```python
from build123d import *

# Parameters (mm, degrees)
SKETCH1_R               = 23.8125
SKETCH1_R_2             = 21.2725
BOSS_EXTRUDE1_DEPTH     = 27.94
SKETCH2_W               = 24.892
SKETCH2_H               = 1.27
SKETCH5_R               = 21.2725
BOSS_EXTRUDE2_DEPTH     = 0.635
CUT_EXTRUDE2_DEPTH      = 37.706625253
CUT_EXTRUDE2_DEPTH_BACK = 37.706625253
SKETCH7_R               = 5.08
BOSS_EXTRUDE7_DEPTH     = 23.495
CUT_EXTRUDE3_DEPTH      = 19.05


with BuildPart() as part:
    # Sketch1 → Boss-Extrude1 (new body)
    with BuildSketch(Plane.XY):
        Circle(SKETCH1_R)
        Circle(SKETCH1_R_2, mode=Mode.SUBTRACT)
    extrude(amount=BOSS_EXTRUDE1_DEPTH)

    # Sketch2 → Cut-Revolve2 (revolve, cut)
    with BuildSketch(Plane(origin=(0, 0, 0), x_dir=(0, 0, -1), z_dir=(1, 0, 0))):
        with Locations((-13.97, 23.1775)):
            Rectangle(SKETCH2_W, SKETCH2_H)
    revolve(axis=Axis((0, 0, 0), (0, 0, 1)), mode=Mode.SUBTRACT)

    # Sketch5 → Boss-Extrude2 (add, symmetric)
    with BuildSketch(Plane.XY.offset(13.97)):
        Circle(SKETCH5_R)
    extrude(amount=BOSS_EXTRUDE2_DEPTH, both=True)

    # Sketch6 → Cut-Extrude2 (cut, two sides: drawn at the far end of the back side and taken through both)
    with BuildSketch(Plane.XY.offset(14.605).offset(-CUT_EXTRUDE2_DEPTH_BACK)):
        with BuildLine():
            Line((0, 5.08), (0, 20.076289255))
            ThreePointArc((0, 20.076289255), (6.203914564, 19.093685719), (11.800546745, 16.242059191))
            Line((11.800546745, 16.242059191), (2.985949082, 4.109806331))
            ThreePointArc((2.985949082, 4.109806331), (1.569806331, 4.831367103), (0, 5.08))
        make_face()
        with BuildLine():
            Line((4.831367103, 1.569806331), (19.093685719, 6.203914564))
            ThreePointArc((19.093685719, 6.203914564), (20.076289255, 0), (19.093685719, -6.203914564))
            Line((19.093685719, -6.203914564), (4.831367103, -1.569806331))
            ThreePointArc((4.831367103, -1.569806331), (5.08, 0), (4.831367103, 1.569806331))
        make_face()
        with BuildLine():
            Line((2.985949082, -4.109806331), (11.800546745, -16.242059191))
            ThreePointArc((11.800546745, -16.242059191), (6.203914564, -19.093685719), (0, -20.076289255))
            Line((0, -20.076289255), (0, -5.08))
            ThreePointArc((0, -5.08), (1.569806331, -4.831367103), (2.985949082, -4.109806331))
        make_face()
        with BuildLine():
            Line((-2.985949082, -4.109806331), (-11.800546745, -16.242059191))
            ThreePointArc((-11.800546745, -16.242059191), (-16.242059191, -11.800546745), (-19.093685719, -6.203914564))
            Line((-19.093685719, -6.203914564), (-4.831367103, -1.569806331))
            ThreePointArc((-4.831367103, -1.569806331), (-4.109806331, -2.985949082), (-2.985949082, -4.109806331))
        make_face()
        with BuildLine():
            Line((-4.831367103, 1.569806331), (-19.093685719, 6.203914564))
            ThreePointArc((-19.093685719, 6.203914564), (-16.242059191, 11.800546745), (-11.800546745, 16.242059191))
            Line((-11.800546745, 16.242059191), (-2.985949082, 4.109806331))
            ThreePointArc((-2.985949082, 4.109806331), (-4.109806331, 2.985949082), (-4.831367103, 1.569806331))
        make_face()
    extrude(amount=CUT_EXTRUDE2_DEPTH + CUT_EXTRUDE2_DEPTH_BACK, mode=Mode.SUBTRACT)

    # Sketch7 → Boss-Extrude7 (add)
    with BuildSketch(Plane.XY.offset(14.605)):
        Circle(SKETCH7_R)
    extrude(amount=BOSS_EXTRUDE7_DEPTH)

    # Sketch8 → Cut-Extrude3 (cut)
    with BuildSketch(Plane.XY.offset(38.1)):
        Polygon((-1.498265311, 3.346047578), (-3.64689486, 0.375487968), (-2.148629549, -2.97055961), (1.498265311, -3.346047578), (3.64689486, -0.375487968), (2.148629549, 2.97055961), align=None)
    extrude(amount=-CUT_EXTRUDE3_DEPTH, mode=Mode.SUBTRACT)


solid = part.part
```
Model file for the job. Use its own axes, mm. A direction names the side the tool comes from. Round coordinates to 2 decimals unless told otherwise and drop trailing zeros. Write each loop counter-clockwise with the first axis right and the second up, starting at its lowest first coordinate (ties: lowest second). Pieces come first, ordered by that corner, then holes. Notation, with made-up numbers: (-30, 9) - (-8, 9) arc R14 ccw to (-8, 18) - close; hole circle Ø7 at (32, 67). An arc over 180 degrees is marked (long way). One line per item, written item: value.
(1) Cut at C-C, the plane y = -18. Give the cut face in (x, z) (3 decimals), plus the area to 3 significant figures.
Values follow:
outline: (-15.59, 0) - (-11.337, 0) - (-11.337, 13.335) - (0, 13.335) - (0, 14.605) - (-11.337, 14.605) - (-11.337, 27.94) - (-15.59, 27.94) - (-15.59, 26.416) - (-13.571, 26.416) - (-13.571, 1.524) - (-15.59, 1.524) - close; (8.891, 13.335) - (11.337, 13.335) - (11.337, 0) - (15.59, 0) - (15.59, 1.524) - (13.571, 1.524) - (13.571, 26.416) - (15.59, 26.416) - (15.59, 27.94) - (11.337, 27.94) - (11.337, 14.605) - (8.891, 14.605) - close
area: 155 mm²
(2) Wall check: probe 1 along Y at (x, z) = (0, 3.25); probe 2 along Z at (x, y) = (-16, -16); probe 3 along Y at (x, z) = (0, 24). Give the ranges that are in metal, low to high.
Values follow:
probe 1: y = -22.54 to -21.27, 21.27 to 22.54
probe 2: z = 0 to 1.52, 26.42 to 27.94
probe 3: y = -22.54 to -21.27, -5.08 to -3.19, 3.19 to 5.08, 21.27 to 22.54
(3) Cut at D-D, the plane x = 15. Give the cut face in (y, z) (3 decimals), plus the area to 3 significant figures.
Values follow:
outline: (-18.494, 0) - (-15.084, 0) - (-15.084, 13.335) - (-4.874, 13.335) - (-4.874, 14.605) - (-15.084, 14.605) - (-15.084, 27.94) - (-18.494, 27.94) - (-18.494, 26.416) - (-16.827, 26.416) - (-16.827, 1.524) - (-18.494, 1.524) - close; (4.874, 13.335) - (15.084, 13.335) - (15.084, 0) - (18.494, 0) - (18.494, 1.524) - (16.827, 1.524) - (16.827, 26.416) - (18.494, 26.416) - (18.494, 27.94) - (15.084, 27.94) - (15.084, 14.605) - (4.874, 14.605) - close
area: 134 mm²
(4) Drop flat-ended pins along their axis: P1, Ø8, axis at x = 9, y = -8, coming from the -Z side (3 decimals); P2, Ø12, axis at y = 9.5, z = 13, coming from the -X side; P3, Ø0.6, axis at y = 12, z = 14.5, coming from the +X side; P4, Ø5, axis at x = -16.5, y = -18.5, coming from the -Z side. Give the stop position or say it passes through.
Values follow:
P1: stops at z = 13.335
P2: stops at x = -22.27
P3: stops at x = 19.27
P4: stops at z = 0
(5) 3-axis set-ups, long thin cutter, end or side, ignore diameter. For faces 4 (the flat face through (0, -13, 14)), 5 (the flat face through (-14, -18, 26.416)), 6 (the cylindrical face through (-16.881, -12.944, 21.179)): which of +Z, -Z, +X, -X, +Y, -Y reach the whole face in a straight line?
Values follow:
face 4: +Z, -Z
face 5: none
face 6: +Z
(6) Cut at B-B, the plane z = 32.5. Give the cut face in (x, y).
Values follow:
outline: circle Ø10.16 at (0, 0); hole (-3.65, 0.38) - (-2.15, -2.97) - (1.5, -3.35) - (3.65, -0.38) - (2.15, 2.97) - (-1.5, 3.35) - close
(7) Two-plate mould, pull along Z, no slides. Class faces 1 (the cylindrical face through (22.006, -4.887, 13.796)), 2 (the flat face through (0, 12, 14)), 3 (the flat face through (0, 0, 13.335)): pulls with the +Z half, pulls with the -Z half, needs draft (parallel to the pull), parting line crosses it, or undercut.
Values follow:
face 1: undercut
face 2: needs draft
face 3: pulls with the -Z half
(8) Cut at A-A, the plane z = 24.5. Give the cut face in (x, y) (1 decimal).
Values follow:
outline: circle Ø45.1 at (0, 0); circle Ø10.2 at (0, 0); hole circle Ø42.5 at (0, 0); hole (-3.6, 0.4) - (-2.1, -3) - (1.5, -3.3) - (3.6, -0.4) - (2.1, 3) - (-1.5, 3.3) - close
